Read the model definition and answer for the solid it produces. Units are mm, in the model's axes. A direction names the side the tool comes from. Coordinates: 2 decimals unless noted, no trailing zeros. Order: outer loops, then holes, each group sorted by start corner. A loop starts at its lowest first (then second) coordinate and runs counter-clockwise, first axis right, second up. Notation, with made-up numbers: (53, 7.5) -> (99, 7.5) arc R25 ccw to (99, 29.5) -> close; hole circle Ø5 at (-22, 17). An arc over 180 degrees is marked (long way). Return JSON: item names as keys, results as strings. Group by question number.
```python
from build123d import *

# Parameters (mm, degrees)
CROQUIS1_R              = 29
SALIENTE_EXTRUIR1_DEPTH = 52
SALIENTE_EXTRUIR2_DEPTH = 10
SALIENTE_EXTRUIR3_START = 3
CROQUIS3_R              = 29
SALIENTE_EXTRUIR3_DEPTH = 3
CROQUIS6_R              = 16
SALIENTE_EXTRUIR4_DEPTH = 0.001
C_PULA1_FACE_RADIUS     = 16
C_PULA1_HEIGHT          = 5
CROQUIS7_R              = 2.05
CORTAR_EXTRUIR1_DEPTH   = 3


with BuildPart() as part:
    # Croquis1 → Saliente-Extruir1 (new body)
    with BuildSketch(Plane(origin=(0, 0, 0), x_dir=(1, 0, 0), z_dir=(0, 1, 0))):
        with Locations(Location((0, 0, 0), (0, 0, 90))):
            Circle(CROQUIS1_R)
    extrude(amount=SALIENTE_EXTRUIR1_DEPTH)

    # Croquis2 → Saliente-Extruir2 (add)
    with BuildSketch(Plane.XZ):
        with BuildLine():
            Line((25.4355, 6), (25.4355, -6))
            Line((25.4355, -6), (26.777981394, -8.18680125))
            ThreePointArc((26.777981394, -8.18680125), (28.0015, 0), (26.777981394, 8.18680125))
            Line((26.777981394, 8.18680125), (25.4355, 6))
        make_face()
        with BuildLine():
            Line((-6, 25.4355), (6, 25.4355))
            Line((6, 25.4355), (8.18680125, 26.777981394))
            ThreePointArc((8.18680125, 26.777981394), (0, 28.0015), (-8.18680125, 26.777981394))
            Line((-8.18680125, 26.777981394), (-6, 25.4355))
        make_face()
        with BuildLine():
            Line((6, -25.4355), (-6, -25.4355))
            Line((-6, -25.4355), (-8.18680125, -26.777981394))
            ThreePointArc((-8.18680125, -26.777981394), (0, -28.0015), (8.18680125, -26.777981394))
            Line((8.18680125, -26.777981394), (6, -25.4355))
        make_face()
        with BuildLine():
            Line((-25.4355, -6), (-25.4355, 6))
            Line((-25.4355, 6), (-26.777981394, 8.18680125))
            ThreePointArc((-26.777981394, 8.18680125), (-28.0015, 0), (-26.777981394, -8.18680125))
            Line((-26.777981394, -8.18680125), (-25.4355, -6))
        make_face()
    extrude(amount=SALIENTE_EXTRUIR2_DEPTH)

    # Croquis3 → Saliente-Extruir3 (add)
    with BuildSketch(Plane.XZ.offset(10).offset(SALIENTE_EXTRUIR3_START)):
        with Locations(Location((0, 0, 0), (0, 0, 270))):
            Circle(CROQUIS3_R)
    extrude(amount=-SALIENTE_EXTRUIR3_DEPTH)

    # Croquis6 → Saliente-Extruir4 (add)
    with BuildSketch(Plane(origin=(0, 52, 0), x_dir=(1, 0, 0), z_dir=(0, 1, 0))):
        with Locations(Location((0, 0, 0), (0, 0, 270))):
            Circle(CROQUIS6_R)
    extrude(amount=SALIENTE_EXTRUIR4_DEPTH)

    # Cúpula1: a dome of height H over a round flat face of radius A is a cap of a sphere of radius (A * A + H * H) / (2 * H)
    c_pula1_r = (C_PULA1_FACE_RADIUS * C_PULA1_FACE_RADIUS + C_PULA1_HEIGHT * C_PULA1_HEIGHT) / (2 * C_PULA1_HEIGHT)
    c_pula1_base = Plane((0, 52.001, 0), z_dir=(0, 1, 0))
    with Locations(c_pula1_base.offset(C_PULA1_HEIGHT - c_pula1_r)):
        c_pula1_ball = Sphere(c_pula1_r, mode=Mode.PRIVATE)
    add(split(c_pula1_ball, bisect_by=c_pula1_base, keep=Keep.TOP, mode=Mode.PRIVATE))

    # Croquis7 → Cortar-Extruir1 (cut)
    with BuildSketch(Plane.XZ.offset(13)):
        with Locations(Location((0, 12, 0), (0, 0, 270))):
            Circle(CROQUIS7_R)
        with Locations(Location((10.392304845, -6, 0), (0, 0, 270))):
            Circle(CROQUIS7_R)
        with Locations(Location((-10.392304845, -6, 0), (0, 0, 270))):
            Circle(CROQUIS7_R)
    extrude(amount=-CORTAR_EXTRUIR1_DEPTH, mode=Mode.SUBTRACT)


solid = part.part
```
1. Which of the six approach directions +Z, -Z, +X, -X, +Y, -Y give full straight-line access (tool end or side, diameter ignored) to faces 1 (the face through (-11.64, -11.521, -4.373)), 2 (the face through (7.08, -4.93, 26.1)), 3 (the face through (0, -10, 0)), 4 (the face through (-25.436, -5, 0))?
2. Find section C-C on y = -5.5. Determine the outline of the cut face in (x, z).
3. For a pull along Y with two mould halves and no side action, classify faces 5 (the face through (12, 52, -12)), 6 (the face through (26.116, -4.93, 7.109)), 7 (the face through (0, 0, 0)), 8 (the face through (0.09, -11.52, 14.05)) as released by +Y, released by -Y, zero draft, split by the parting line, or undercut.
4. Given pin 1 (12 mm diameter, centred on y = 35.5, z = 4.5, fed in from -X); pin 2 (4 mm diameter, centred on y = 16.5, z = 22.5, fed in from -X); pin 3 (17.5 mm diameter, centred on x = 0.5, z = -9.5, fed in from +Y); pin 4 (4 mm diameter, centred on y = -3, z = 12, fed in from -X), each flat-ended and moving along its own axis, determine where each tip first touches the part or whether it passes through.
5. Find section B-B on z = -21. Determine the outline of the cut face in (x, y).
6. Find section D-D on x = 9.5. Give the number of separate pieces and of enclosed holes in the cut face, and give its area (3 significant figures).
7. Straight lines are drawn through the part: L1, parallel to Y at x = -12.5, z = 24; L2, parallel to X at y = -11.35, z = -6; L3, parallel to Y at x = 1, z = -11. For each, find the intervals that lie inside material, in ascending order.
Result:
{
 "1": {"face 1": "-Y", "face 2": "+X", "face 3": "none", "face 4": "+Z, -Z"},
 "2": {"outline": "(-26.78, -8.19) -> (-25.44, -6) -> (-25.44, 6) -> (-26.78, 8.19) arc R28 ccw to start; (-8.19, -26.78) arc R28 ccw to (8.19, -26.78) -> (6, -25.44) -> (-6, -25.44) -> close; (-8.19, 26.78) -> (-6, 25.44) -> (6, 25.44) -> (8.19, 26.78) arc R28 ccw to start; (25.44, -6) -> (26.78, -8.19) arc R28 ccw to (26.78, 8.19) -> (25.44, 6) -> close"},
 "3": {"face 5": "released by +Y", "face 6": "undercut", "face 7": "undercut", "face 8": "zero draft"},
 "4": {"pin 1": "x = -29", "pin 2": "x = -20.51", "pin 3": "y = 56.99", "pin 4": "through"},
 "5": {"outline": "(-20, -13) -> (20, -13) -> (20, -10) -> (-20, -10) -> close; (-20, 0) -> (20, 0) -> (20, 52) -> (-20, 52) -> close"},
 "6": {"separate pieces": "3", "enclosed holes": "0", "area": "3,060 mm^2"},
 "7": {"L1": "-13 to -10, 0 to 52", "L2": "-28.37 to -12.44, -8.34 to 8.34, 12.44 to 28.37", "L3": "-13 to -10, 0 to 54.74"}
}
